Read the model definition and answer for the solid it produces. Units are mm, in the model's axes. A direction names the side the tool comes from. Coordinates: 2 decimals unless noted, no trailing zeros. Write each loop counter-clockwise with the first axis right and the second up, starting at its lowest first coordinate (ties: lowest second). Pieces come first, ordered by that corner, then holes. Notation, with made-up numbers: (43.5, 4.5) -> (50.5, 4.5) arc R15 cw to (50.5, 21.5) -> close; hole circle Ø4 at (-17.75, -17). An arc over 180 degrees is marked (long way). Write item = value, one per line. Start each with the question number.
1) Section A-A (x = -12.5) is taken. Determine the outline of the cut face in (y, z), plus the area to 3 significant figures.
2) Find the intervals of material crossed by line 1 along X through (y, z) = (6, 7.25); line 2 along Y through (x, z) = (-19, 3.75); line 3 along Y through (x, z) = (-2, 2), in increasing order. Write a range as from..to.
3) Section B-B (y = -9.5) is taken. Determine the outline of the cut face in (x, z).
4) Flat-ended cylindrical pins translate along their axes: pin 1 Ø1.5 at (x, z) = (-9, 3.5) entering from +Y; pin 2 Ø1.8 at (y, z) = (-8, 5.5) entering from +X; pin 3 Ø2 at (y, z) = (-20.5, 5.5) entering from +X; pin 4 Ø2 at (x, z) = (-4, 8) entering from -Y. Find the tip coordinate at first contact, or state that the pin passes through.
5) A tool of negligible diameter and unlimited length cuts with its end or side. For faces 1 (the face through (4.084, -20.809, 5.042)), 2 (the face through (-2.201, 3.043, 0.792)), 3 (the face through (3.161, 2.984, 0.792)), 4 (the face through (-5.37, -28.336, 8.764)), from which of +Z, -Z, +X, -X, +Y, -Y can it reach the whole face along a straight path? Write none if from no direction.
6) For a pull along Y with two mould halves and no side action, classify faces 5 (the face through (-27, -9, 10)), 6 (the face through (-14, 20.695, 5)), 7 (the face through (-5.46, 9.815, 1.236)) as released by +Y, released by -Y, zero draft, split by the parting line, or undercut.
from build123d import *

# Parameters (mm, degrees)
F0_W         = 10
F0_H         = 10
F1_DEPTH     = 10
F2_R         = 4.99999
F3_R         = 15
F4_T1_DEPTH  = 30
F4_T3_DEPTH  = 10
F4_T5_DEPTH  = 1e-05
F4_T7_DEPTH  = 2e-05
F4_T9_DEPTH  = 2e-05
F4_T11_DEPTH = 10.00002
F4_T13_DEPTH = 30.00002
F4_T15_DEPTH = 2e-05
F4_T17_DEPTH = 1e-05
F4_T20_ANGLE = 90
F4_T22_ANGLE = 90
F4_T24_ANGLE = 90
F4_T26_ANGLE = 90
F4_T28_ANGLE = 90
F4_T30_ANGLE = 90
F4_T32_ANGLE = 90
F4_T34_ANGLE = 90
F4_T36_ANGLE = 90
F4_T38_ANGLE = 90
F4_T40_ANGLE = 90
F4_T42_ANGLE = 90
F4_T44_ANGLE = 90
F4_T46_ANGLE = 90
F4_T48_ANGLE = 90
F4_T50_ANGLE = 90
F4_T52_ANGLE = 90
F4_T54_ANGLE = 90
F4_T56_ANGLE = 90
F4_T58_ANGLE = 90
F4_T60_ANGLE = 90
F4_T62_ANGLE = 90
F4_T64_ANGLE = 90
F4_T66_ANGLE = 90


# Not quite as in the source:
# - a fillet or chamfer that OpenCascade refuses, or shapes differently, is made with other operations: its cross-section is extruded or revolved along the edge and cut away or added
# - a fillet or chamfer is up to 0.001 mm smaller than in the source, because OpenCascade refuses the exact size


with BuildPart() as f1:
    # F0 (on Top) → F1 (new body)
    with BuildSketch(Plane.XY):
        Polygon((-4.4905686265, 20.6948744461), (-34.4905686265, 20.6948744461), (-34.4905686265, 10.6948744461), (-24.4905686265, 10.6948744461), (-4.4905686265, 10.6948744461), align=None)
        Polygon((5.5094313735, 20.6948744461), (-4.4905686265, 20.6948744461), (-4.4905686265, 10.6948744461), (-4.4905686265, 0.6948744461), (5.5094313735, 0.6948744461), align=None)
        with Locations((0.5094313735, -24.3051255539)):
            Rectangle(F0_W, F0_H)
        Polygon((-24.4905686265, 10.6948744461), (-34.4905686265, 10.6948744461), (-34.4905686265, -39.3051255539), (-24.4905686265, -39.3051255539), (-24.4905686265, -29.3051255539), align=None)
        Polygon((-4.4905686265, -29.3051255539), (-24.4905686265, -29.3051255539), (-24.4905686265, -39.3051255539), (5.5094313735, -39.3051255539), (5.5094313735, -29.3051255539), align=None)
    extrude(amount=F1_DEPTH)

    # F2 (radius 5 in the source; OpenCascade refuses exactly that, so slightly less here)
    f2_edges = [f1.edges().sort_by_distance(p)[0] for p in [
        (5.509431, 0.694874, 5),
        (-4.490569, 0.694874, 5),
        (-4.490569, 10.694874, 5),
        (5.509431, -19.305126, 5),
        (-4.490569, -19.305126, 5),
        (-24.490569, 10.694874, 5),
        (-24.490569, -29.305126, 5),
        (-4.490569, -29.305126, 5),
    ]]
    fillet(f2_edges, radius=F2_R)

    # F3
    f3_edges = [f1.edges().sort_by_distance(p)[0] for p in [
        (-34.490569, 20.694874, 5),
        (5.509431, 20.694874, 5),
        (5.509431, -39.305126, 5),
        (-34.490569, -39.305126, 5),
    ]]
    fillet(f3_edges, radius=F3_R)

    # F4: chamfer of 2 on 2 edges, made by hand

    # F4_s2 → F4_t1 (cut)
    with BuildSketch(Plane.XZ.offset(-5.6948744461)):
        Polygon((-32.4905686265, 10), (-34.4905686265, 8), (-34.4905686265, 10), align=None)
        Polygon((-32.4905686265, 0), (-34.4905686265, 2), (-34.4905686265, 0), align=None)
    extrude(amount=F4_T1_DEPTH, mode=Mode.SUBTRACT)

    # F4_s4 → F4_t3 (cut)
    with BuildSketch(Plane.YZ.offset(-19.4905686265)):
        Polygon((-37.3051255539, 0), (-39.3051255539, 2), (-39.3051255539, 0), align=None)
        Polygon((18.6948744461, 0), (20.6948744461, 2), (20.6948744461, 0), align=None)
        Polygon((-37.3051255539, 10), (-39.3051255539, 8), (-39.3051255539, 10), align=None)
        Polygon((18.6948744461, 10), (20.6948744461, 8), (20.6948744461, 10), align=None)
    extrude(amount=F4_T3_DEPTH, mode=Mode.SUBTRACT)

    # F4_s6 → F4_t5 (cut)
    with BuildSketch(Plane.XZ.offset(24.3051155539)):
        Polygon((5.5094313735, 2), (3.5094313735, 0), (5.5094313735, 0), align=None)
        Polygon((5.5094313735, 8), (3.5094313735, 10), (5.5094313735, 10), align=None)
    extrude(amount=F4_T5_DEPTH, mode=Mode.SUBTRACT)

    # F4_s8 → F4_t7 (cut)
    with BuildSketch(Plane.YZ.offset(0.5094213735)):
        Polygon((-21.3051255539, 0), (-19.3051255539, 2), (-19.3051255539, 0), align=None)
        Polygon((2.6948744461, 0), (0.6948744461, 2), (0.6948744461, 0), align=None)
        Polygon((-21.3051255539, 10), (-19.3051255539, 8), (-19.3051255539, 10), align=None)
        Polygon((2.6948744461, 10), (0.6948744461, 8), (0.6948744461, 10), align=None)
    extrude(amount=F4_T7_DEPTH, mode=Mode.SUBTRACT)

    # F4_s10 → F4_t9 (cut)
    with BuildSketch(Plane.XZ.offset(24.3051155539)):
        Polygon((-2.4905686265, 0), (-4.4905686265, 2), (-4.4905686265, 0), align=None)
        Polygon((-2.4905686265, 10), (-4.4905686265, 8), (-4.4905686265, 10), align=None)
    extrude(amount=F4_T9_DEPTH, mode=Mode.SUBTRACT)

    # F4_s12 → F4_t11 (cut)
    with BuildSketch(Plane.YZ.offset(-19.4905786265)):
        Polygon((-31.3051255539, 0), (-29.3051255539, 2), (-29.3051255539, 0), align=None)
        Polygon((12.6948744461, 0), (10.6948744461, 2), (10.6948744461, 0), align=None)
        Polygon((-31.3051255539, 10), (-29.3051255539, 8), (-29.3051255539, 10), align=None)
        Polygon((12.6948744461, 10), (10.6948744461, 8), (10.6948744461, 10), align=None)
    extrude(amount=F4_T11_DEPTH, mode=Mode.SUBTRACT)

    # F4_s14 → F4_t13 (cut)
    with BuildSketch(Plane.XZ.offset(-5.6948844461)):
        Polygon((-26.4905686265, 0), (-24.4905686265, 2), (-24.4905686265, 0), align=None)
        Polygon((-26.4905686265, 10), (-24.4905686265, 8), (-24.4905686265, 10), align=None)
    extrude(amount=F4_T13_DEPTH, mode=Mode.SUBTRACT)

    # F4_s16 → F4_t15 (cut)
    with BuildSketch(Plane.XZ.offset(-5.6948844461)):
        Polygon((-2.4905686265, 0), (-4.4905686265, 2), (-4.4905686265, 0), align=None)
        Polygon((-2.4905686265, 10), (-4.4905686265, 8), (-4.4905686265, 10), align=None)
    extrude(amount=F4_T15_DEPTH, mode=Mode.SUBTRACT)

    # F4_s18 → F4_t17 (cut)
    with BuildSketch(Plane.XZ.offset(-5.6948744461)):
        Polygon((3.5094313735, 0), (5.5094313735, 2), (5.5094313735, 0), align=None)
        Polygon((3.5094313735, 10), (5.5094313735, 8), (5.5094313735, 10), align=None)
    extrude(amount=F4_T17_DEPTH, mode=Mode.SUBTRACT)

    # F4_s19 → F4_t20 (revolve, cut)
    with BuildSketch(Plane.XZ.offset(-5.6948744461)):
        Polygon((-32.4905686265, 0), (-34.4905686265, 2), (-34.4905686265, 0), align=None)
    revolve(axis=Axis((-19.4905686265, 5.6948744461, 0), (0, 0, -1)), revolution_arc=F4_T20_ANGLE, mode=Mode.SUBTRACT)

    # F4_s21 → F4_t22 (revolve, cut)
    with BuildSketch(Plane.YZ.offset(-19.4905686265)):
        Polygon((-37.3051255539, 0), (-39.3051255539, 2), (-39.3051255539, 0), align=None)
    revolve(axis=Axis((-19.4905686265, -24.3051255539, 0), (0, 0, -1)), revolution_arc=F4_T22_ANGLE, mode=Mode.SUBTRACT)

    # F4_s23 → F4_t24 (revolve, cut)
    with BuildSketch(Plane.XZ.offset(24.3051255539)):
        Polygon((3.5094313735, 0), (5.5094313735, 2), (5.5094313735, 0), align=None)
    revolve(axis=Axis((-9.4905686265, -24.3051255539, 0), (0, 0, -1)), revolution_arc=F4_T24_ANGLE, mode=Mode.SUBTRACT)

    # F4_s25 → F4_t26 (revolve, cut)
    with BuildSketch(Plane.XZ.offset(24.3051155539)):
        Polygon((3.5094313735, 0), (5.5094313735, 2), (5.5094313735, 0), align=None)
    revolve(axis=Axis((0.5094413735, -24.3051155539, 0), (0, 0, 1)), revolution_arc=F4_T26_ANGLE, mode=Mode.SUBTRACT)

    # F4_s27 → F4_t28 (revolve, cut)
    with BuildSketch(Plane.YZ.offset(0.5094213735)):
        Polygon((-21.3051255539, 0), (-19.3051255539, 2), (-19.3051255539, 0), align=None)
    revolve(axis=Axis((0.5094213735, -24.3051155539, 0), (0, 0, 1)), revolution_arc=F4_T28_ANGLE, mode=Mode.SUBTRACT)

    # F4_s29 → F4_t30 (revolve, cut)
    with BuildSketch(Plane.XZ.offset(24.3051355539)):
        Polygon((-2.4905686265, 0), (-4.4905686265, 2), (-4.4905686265, 0), align=None)
    revolve(axis=Axis((-9.4905586265, -24.3051355539, 0), (0, 0, -1)), revolution_arc=F4_T30_ANGLE, mode=Mode.SUBTRACT)

    # F4_s31 → F4_t32 (revolve, cut)
    with BuildSketch(Plane.YZ.offset(-19.4905786265)):
        Polygon((-31.3051255539, 0), (-29.3051255539, 2), (-29.3051255539, 0), align=None)
    revolve(axis=Axis((-19.4905786265, -24.3051355539, 0), (0, 0, -1)), revolution_arc=F4_T32_ANGLE, mode=Mode.SUBTRACT)

    # F4_s33 → F4_t34 (revolve, cut)
    with BuildSketch(Plane.XZ.offset(-5.6948844461)):
        Polygon((-26.4905686265, 0), (-24.4905686265, 2), (-24.4905686265, 0), align=None)
    revolve(axis=Axis((-19.4905786265, 5.6948844461, 0), (0, 0, -1)), revolution_arc=F4_T34_ANGLE, mode=Mode.SUBTRACT)

    # F4_s35 → F4_t36 (revolve, cut)
    with BuildSketch(Plane.YZ.offset(-9.4905586265)):
        Polygon((12.6948744461, 0), (10.6948744461, 2), (10.6948744461, 0), align=None)
    revolve(axis=Axis((-9.4905586265, 5.6948844461, 0), (0, 0, -1)), revolution_arc=F4_T36_ANGLE, mode=Mode.SUBTRACT)

    # F4_s37 → F4_t38 (revolve, cut)
    with BuildSketch(Plane.XZ.offset(-5.6948644461)):
        Polygon((-2.4905686265, 0), (-4.4905686265, 2), (-4.4905686265, 0), align=None)
    revolve(axis=Axis((0.5094213735, 5.6948644461, 0), (0, 0, 1)), revolution_arc=F4_T38_ANGLE, mode=Mode.SUBTRACT)

    # F4_s39 → F4_t40 (revolve, cut)
    with BuildSketch(Plane.YZ.offset(0.5094413735)):
        Polygon((2.6948744461, 0), (0.6948744461, 2), (0.6948744461, 0), align=None)
    revolve(axis=Axis((0.5094413735, 5.6948644461, 0), (0, 0, 1)), revolution_arc=F4_T40_ANGLE, mode=Mode.SUBTRACT)

    # F4_s41 → F4_t42 (revolve, cut)
    with BuildSketch(Plane.YZ.offset(-9.4905686265)):
        Polygon((18.6948744461, 0), (20.6948744461, 2), (20.6948744461, 0), align=None)
    revolve(axis=Axis((-9.4905686265, 5.6948744461, 0), (0, 0, -1)), revolution_arc=F4_T42_ANGLE, mode=Mode.SUBTRACT)

    # F4_s43 → F4_t44 (revolve, cut)
    with BuildSketch(Plane.XZ.offset(-5.6948744461)):
        Polygon((-32.4905686265, 10), (-34.4905686265, 8), (-34.4905686265, 10), align=None)
    revolve(axis=Axis((-19.4905686265, 5.6948744461, 10), (0, 0, -1)), revolution_arc=F4_T44_ANGLE, mode=Mode.SUBTRACT)

    # F4_s45 → F4_t46 (revolve, cut)
    with BuildSketch(Plane.YZ.offset(-19.4905686265)):
        Polygon((-37.3051255539, 10), (-39.3051255539, 8), (-39.3051255539, 10), align=None)
    revolve(axis=Axis((-19.4905686265, -24.3051255539, 10), (0, 0, -1)), revolution_arc=F4_T46_ANGLE, mode=Mode.SUBTRACT)

    # F4_s47 → F4_t48 (revolve, cut)
    with BuildSketch(Plane.XZ.offset(24.3051255539)):
        Polygon((5.5094313735, 8), (3.5094313735, 10), (5.5094313735, 10), align=None)
    revolve(axis=Axis((-9.4905686265, -24.3051255539, 10), (0, 0, -1)), revolution_arc=F4_T48_ANGLE, mode=Mode.SUBTRACT)

    # F4_s49 → F4_t50 (revolve, cut)
    with BuildSketch(Plane.XZ.offset(24.3051155539)):
        Polygon((5.5094313735, 8), (3.5094313735, 10), (5.5094313735, 10), align=None)
    revolve(axis=Axis((0.5094413735, -24.3051155539, 10), (0, 0, 1)), revolution_arc=F4_T50_ANGLE, mode=Mode.SUBTRACT)

    # F4_s51 → F4_t52 (revolve, cut)
    with BuildSketch(Plane.YZ.offset(0.5094213735)):
        Polygon((-21.3051255539, 10), (-19.3051255539, 8), (-19.3051255539, 10), align=None)
    revolve(axis=Axis((0.5094213735, -24.3051155539, 10), (0, 0, 1)), revolution_arc=F4_T52_ANGLE, mode=Mode.SUBTRACT)

    # F4_s53 → F4_t54 (revolve, cut)
    with BuildSketch(Plane.XZ.offset(24.3051355539)):
        Polygon((-2.4905686265, 10), (-4.4905686265, 8), (-4.4905686265, 10), align=None)
    revolve(axis=Axis((-9.4905586265, -24.3051355539, 10), (0, 0, -1)), revolution_arc=F4_T54_ANGLE, mode=Mode.SUBTRACT)

    # F4_s55 → F4_t56 (revolve, cut)
    with BuildSketch(Plane.YZ.offset(-19.4905786265)):
        Polygon((-31.3051255539, 10), (-29.3051255539, 8), (-29.3051255539, 10), align=None)
    revolve(axis=Axis((-19.4905786265, -24.3051355539, 10), (0, 0, -1)), revolution_arc=F4_T56_ANGLE, mode=Mode.SUBTRACT)

    # F4_s57 → F4_t58 (revolve, cut)
    with BuildSketch(Plane.XZ.offset(-5.6948844461)):
        Polygon((-26.4905686265, 10), (-24.4905686265, 8), (-24.4905686265, 10), align=None)
    revolve(axis=Axis((-19.4905786265, 5.6948844461, 10), (0, 0, -1)), revolution_arc=F4_T58_ANGLE, mode=Mode.SUBTRACT)

    # F4_s59 → F4_t60 (revolve, cut)
    with BuildSketch(Plane.YZ.offset(-9.4905586265)):
        Polygon((12.6948744461, 10), (10.6948744461, 8), (10.6948744461, 10), align=None)
    revolve(axis=Axis((-9.4905586265, 5.6948844461, 10), (0, 0, -1)), revolution_arc=F4_T60_ANGLE, mode=Mode.SUBTRACT)

    # F4_s61 → F4_t62 (revolve, cut)
    with BuildSketch(Plane.XZ.offset(-5.6948644461)):
        Polygon((-2.4905686265, 10), (-4.4905686265, 8), (-4.4905686265, 10), align=None)
    revolve(axis=Axis((0.5094213735, 5.6948644461, 10), (0, 0, 1)), revolution_arc=F4_T62_ANGLE, mode=Mode.SUBTRACT)

    # F4_s63 → F4_t64 (revolve, cut)
    with BuildSketch(Plane.YZ.offset(0.5094413735)):
        Polygon((2.6948744461, 10), (0.6948744461, 8), (0.6948744461, 10), align=None)
    revolve(axis=Axis((0.5094413735, 5.6948644461, 10), (0, 0, 1)), revolution_arc=F4_T64_ANGLE, mode=Mode.SUBTRACT)

    # F4_s65 → F4_t66 (revolve, cut)
    with BuildSketch(Plane.YZ.offset(-9.4905686265)):
        Polygon((18.6948744461, 10), (20.6948744461, 8), (20.6948744461, 10), align=None)
    revolve(axis=Axis((-9.4905686265, 5.6948744461, 10), (0, 0, -1)), revolution_arc=F4_T66_ANGLE, mode=Mode.SUBTRACT)


solid = f1.part
Answer key:
q1.outline = (-39.31, 2) -> (-37.31, 0) -> (-31.31, 0) -> (-29.31, 2) -> (-29.31, 8) -> (-31.31, 10) -> (-37.31, 10) -> (-39.31, 8) -> close; (10.69, 2) -> (12.69, 0) -> (18.69, 0) -> (20.69, 2) -> (20.69, 8) -> (18.69, 10) -> (12.69, 10) -> (10.69, 8) -> close
q1.area = 184 mm^2
q2.line_1 = -34.49..-24.48, -4.5..5.51
q2.line_2 = -39.31..-29.31, 10.69..20.69
q2.line_3 = -37.3..-19.98, 1.37..18.69
q3.outline = (-34.49, 2) -> (-32.49, 0) -> (-26.49, 0) -> (-24.49, 2) -> (-24.49, 8) -> (-26.49, 10) -> (-32.49, 10) -> (-34.49, 8) -> close
q4.pin_1 = 20.69
q4.pin_2 = -24.49
q4.pin_3 = 4.65
q4.pin_4 = -38.62
q5.face_1 = +Z, -Z, +X
q5.face_2 = -Z
q5.face_3 = -Z, +X
q5.face_4 = +Z
q6.face_5 = zero draft
q6.face_6 = released by +Y
q6.face_7 = undercut
